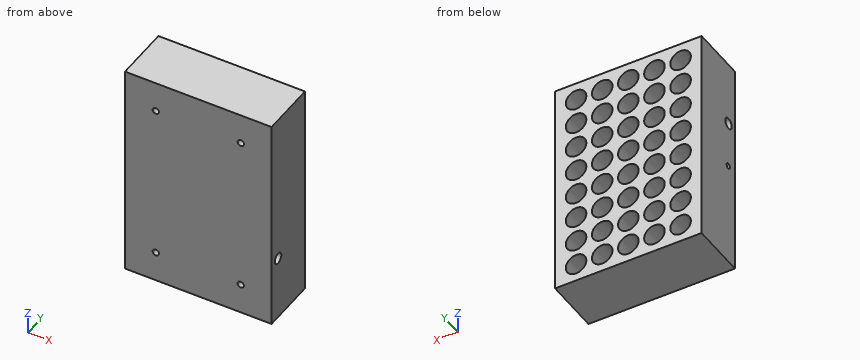
Autodesk Inventor part; units mm, degrees
ref_plane "YZ Plane" through (0, 0, 0) normal (1, 0, 0) x (0, 1, 0)
ref_plane "XZ Plane" through (0, 0, 0) normal (0, 1, 0) x (-1, 0, 0)
ref_plane "XY Plane" through (0, 0, 0) normal (0, 0, 1) x (1, 0, 0)
sketch "Sketch1" plane through (0, 0, 0) normal (0, 1, 0) x (-1, 0, 0)
  line L0 (0, 0) -> (85.48, 0)
  line L1 (85.48, 0) -> (85.48, -127.76)
  line L2 (85.48, -127.76) -> (0, -127.76)
  line L3 (0, -127.76) -> (0, 0)
  line L4 (85.48, 0) -> (67.5195, -17.9605)
  line L5 (85.48, 0) -> (110.88, 0) construction
  line L6 (0, 0) -> (17.9605, -17.9605)
  line L7 (85.48, -127.76) -> (67.5195, -109.7995)
  line L8 (85.48, -127.76) -> (110.88, -127.76) construction
  line L9 (0, -127.76) -> (17.9605, -109.7995)
  line L10 (0, -127.76) -> (25.4, -127.76) construction
  dimension "d0" = 85.48
  dimension "d1" = 127.76
  dimension "d2" = 25.4
  dimension "d3" = 135
  dimension "d4" = 25.4
  dimension "d5" = 25.4
  dimension "d6" = 135
  dimension "d7" = 25.4
  dimension "d8" = 45
extrude "Extrusion1" add sketch "Sketch1" along normal blind 32.7
sketch "Sketch2" plane through (0, 0, 0) normal (0, -1, 0) x (1, 0, 0)
  line L0 (-85.48, 0) -> (0, 0)
  line L1 (0, 0) -> (-17.9605, -17.9605)
  line L2 (0, 0) -> (25.4, 0) construction
  line L3 (0, 0) -> (0, -127.76)
  line L4 (0, -127.76) -> (-17.9605, -109.7995)
  line L5 (0, -127.76) -> (25.4, -127.76) construction
  line L6 (-85.48, -127.76) -> (-85.48, 0)
  line L7 (-85.48, 0) -> (-67.5195, -17.9605)
  line L8 (-85.48, 0) -> (-60.08, 0) construction
  line L9 (0, -127.76) -> (-85.48, -127.76)
  line L10 (-85.48, -127.76) -> (-67.5195, -109.7995)
  line L11 (-85.48, -127.76) -> (-60.08, -127.76) construction
  dimension "d11" = 25.4
  dimension "d12" = 135
  dimension "d13" = 25.4
  dimension "d14" = 135
  dimension "d15" = 25.4
  dimension "d16" = 45
  dimension "d17" = 25.4
  dimension "d18" = 45
hole "Hole1" at (-17.9605, 0, -17.9605) at (-67.5195, 0, -17.9605) at (-67.5195, 0, -109.7995) at (-17.9605, 0, -109.7995) direction (0, 1, 0) diameter 3.683 depth 9.525 tip angle 118
sketch "Sketch4" plane through (0, 32.7, 0) normal (0, 1, 0) x (1, 0, 0)
  line L0 (0, -1.0521) -> (19.05, -1.0521) construction
  line L1 (0, 0) -> (0, 127.76)
  line L2 (0, 18.3507) -> (0, 0)
  line L3 (0, 0) -> (-18.7946, 0)
  line L4 (0, 0) -> (-12.2682, 0)
  line L5 (-12.2682, 0) -> (-12.2682, 10.541)
  line L6 (-12.2682, 10.541) -> (0, 10.541)
  line L7 (0, 10.541) -> (0, 0)
  dimension "d41" = 12.2682
  dimension "d42" = 10.541
hole "Hole2" at (-12.2682, 32.7, -10.541) direction (0, -1, 0) diameter 12 depth 20
pattern_linear "Rectangular Pattern1" count 5 spacing 15.24 along (-1, 0, 0) count 8 spacing 15.24 along (0, 0, -1) of "Hole2"
sketch "Sketch5" plane through (-85.48, 0, -127.76) normal (-1, 0, 0) x (0, 0, 1)
  line L0 (127.76, 0) -> (127.76, 32.7)
  line L1 (127.76, 0) -> (89.66, 0)
  line L2 (89.66, 0) -> (89.66, 6.35)
  line L3 (89.66, 6.35) -> (127.76, 6.35)
  line L4 (127.76, 6.35) -> (127.76, 0)
  line L5 (62.646, 6.35) -> (127.76, 6.35)
  line L6 (127.76, 6.35) -> (127.76, 0)
  line L7 (127.76, 0) -> (62.646, 0)
  line L8 (62.646, 0) -> (62.646, 6.35)
  dimension "d43" = 38.1
  dimension "d44" = 6.35
hole "Hole3" at (-85.48, 6.35, -38.1) direction (1, 0, 0) diameter 6.35 depth 31.75 tip angle 118
sketch "Sketch6" plane through (-85.48, 0, -127.76) normal (-1, 0, 0) x (0, 0, 1)
  line L0 (61.854, 6.5465) -> (127.76, 6.5465)
  line L1 (127.76, 6.5465) -> (127.76, 0.1965)
  line L2 (127.76, 0.1965) -> (61.854, 0.1965)
  line L3 (61.854, 0.1965) -> (61.854, 6.5465)
  point P0 (127.76, 0)
  dimension "d52" = 6.35
hole "Hole4" at (-85.48, 6.5465, -65.906) direction (1, 0, 0) diameter 3.175 depth 50.8 tip angle 118
sketch "Sketch7" plane through (0, 0, 0) normal (1, 0, 0) x (0, 0, -1)
  line L0 (127.76, 0) -> (0, 0)
  line L1 (127.76, 0) -> (89.66, 0)
  line L2 (89.66, 0) -> (89.66, 6.35)
  line L3 (89.66, 6.35) -> (127.76, 6.35)
  line L4 (127.76, 6.35) -> (127.76, 0)
  dimension "d60" = 38.1
  dimension "d61" = 6.35
hole "Hole5" at (0, 6.35, -89.66) direction (-1, 0, 0) diameter 6.35 depth 31.75 tip angle 118
properties part number "Thermal_topplate_1mL"
The model under review builds one solid part; all positions refer to its coordinate system, in mm. Give positions to 0.01 mm unless a question says otherwise; leave off trailing zeros. Loops run counter-clockwise (first coordinate to the right, second up) from the corner with the lowest first, then second, coordinate; pieces in that order, holes last. Notation, with made-up numbers: (31.5, -15.5) -> (60.5, -15.5) arc R22 ccw to (60.5, 11.5) -> close; hole circle Ø2 at (45.25, 7). An arc over 180 degrees is marked (long way). Answer as a JSON object with one key per item and string values. Group by question number.
Q1. Take a section at B-B (y = 24.5). State how many separate pieces and enclosed holes the cut face has, plus the area to 3 significant figures.
Q2. Take a section at A-A (z = -61). Write out the cut boundary in (x, y), plus the area to 3 significant figures.
Q3. Insertion check: pin 1 (2 mm diameter, centred on x = -35.5, y = 9, fed in from +Z); pin 2 (9.5 mm diameter, centred on x = -12.27, z = -71.5, fed in from +Y); pin 3 (3.5 mm diameter, centred on x = -17.96, z = -109.8, fed in from -Y). Each pin has a flat end and moves straight along its axis. Give the tip position at first contact, or say it passes through.
Q4. Wall thickness on line 1 along X through (y, z) = (6, -110); line 2 along X through (y, z) = (30, -41); line 3 along Z through (x, y) = (-72, 6.5): over which ranges is each line inside the solid? List them lowest first.
Answer below:
{
 "1": {"separate pieces": "1", "enclosed holes": "40", "area": "6,400 mm2"},
 "2": {"outline": "(-85.48, 0) -> (0, 0) -> (0, 32.7) -> (-8.59, 32.7) -> (-8.59, 12.7) -> (-15.95, 12.7) -> (-15.95, 32.7) -> (-23.83, 32.7) -> (-23.83, 12.7) -> (-31.19, 12.7) -> (-31.19, 32.7) -> (-39.07, 32.7) -> (-39.07, 12.7) -> (-46.43, 12.7) -> (-46.43, 32.7) -> (-54.31, 32.7) -> (-54.31, 12.7) -> (-61.67, 12.7) -> (-61.67, 32.7) -> (-69.55, 32.7) -> (-69.55, 12.7) -> (-76.91, 12.7) -> (-76.91, 32.7) -> (-85.48, 32.7) -> close", "area": "2,060 mm2"},
 "3": {"pin 1": "stops at z = 0", "pin 2": "stops at y = 12.7", "pin 3": "stops at y = 9.58"},
 "4": {"line 1": "x = -85.48 to -69.35, -65.69 to -19.79, -16.13 to 0", "line 2": "x = -85.48 to -79.23, -67.23 to -63.99, -51.99 to -48.75, -36.75 to -33.51, -21.51 to -18.27, -6.27 to 0", "line 3": "z = -127.76 to -67.49, -64.32 to -41.27, -34.93 to 0"}
}
